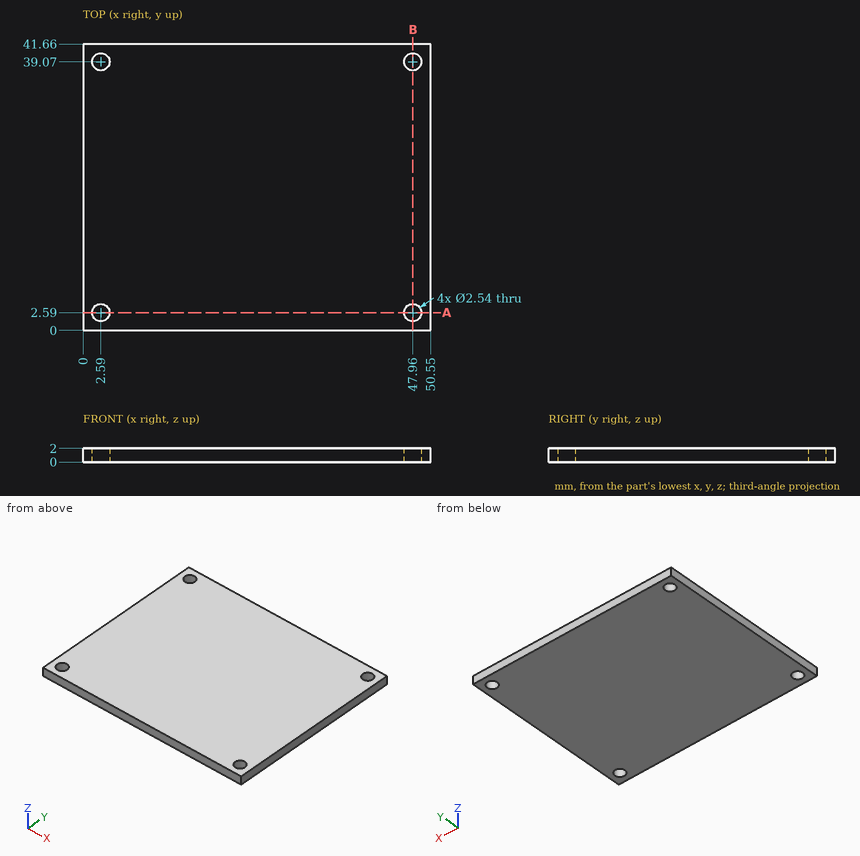
Study the drawing (mm; zero at the part's minimum x, y, z) and answer. Give positions to 0.01 mm unless a question says otherwise; leave off trailing zeros. Order: outer loops, then holes, each group sorted by start corner. A loop starts at its lowest first (then second) coordinate and runs counter-clockwise, first axis right, second up. Notation, with made-up numbers: (29.5, -31.75) - (36.5, -31.75) arc R15 cw to (36.5, -16.75) - close; hole circle Ø7 at (13.5, 22). An arc over 180 degrees is marked (long way). Answer in a Markdown table with one row per item. Add a question column.
Q1. The part is cut by section A-A (y = 2.59). Determine the outline of the cut face in (x, z).
Q2. Find the intervals of material crossed by line 1 along Y through (x, z) = (47.96, 0.9); line 2 along X through (y, z) = (39, 1.4); line 3 along X through (y, z) = (38, 1.5), in increasing order. Write a range as [from, to].
Q3. Given P1, Ø2, axis at x = 47.96, y = 39.07, coming from the -Z side (3 decimals), flat-ended and moving along its own axis, determine where the tip first touches the part or whether it passes through.
Q4. The part is cut by section B-B (x = 47.96). Determine the outline of the cut face in (y, z), then the cut area to 3 significant figures.
Determined:
| question | item | result |
|---|---|---|
| 1 | outline | (0, 0) - (1.32, 0) - (1.32, 2) - (0, 2) - close; (3.86, 0) - (46.69, 0) - (46.69, 2) - (3.86, 2) - close; (49.23, 0) - (50.55, 0) - (50.55, 2) - (49.23, 2) - close |
| 2 | line 1 | y = [0, 1.32], [3.86, 37.8], [40.34, 41.66] |
| 2 | line 2 | x = [0, 1.32], [3.86, 46.69], [49.23, 50.55] |
| 2 | line 3 | x = [0, 1.91], [3.27, 47.28], [48.64, 50.55] |
| 3 | P1 | passes through |
| 4 | outline | (0, 0) - (1.32, 0) - (1.32, 2) - (0, 2) - close; (3.86, 0) - (37.8, 0) - (37.8, 2) - (3.86, 2) - close; (40.34, 0) - (41.66, 0) - (41.66, 2) - (40.34, 2) - close |
| 4 | area | 73.2 mm² |
